Build history of the part. All positions in model axes, mm. Round coordinates to 2 decimals unless told otherwise and drop trailing zeros. Write each loop counter-clockwise with the first axis right and the second up, starting at its lowest first coordinate (ties: lowest second). Pieces come first, ordered by that corner, then holes. Notation, with made-up numbers: (51.5, 28.25) - (99.5, 28.25) arc R14 cw to (99.5, 47.25) - close; hole circle Ø6 at (26.5, 46.25). An arc over 180 degrees is marked (long way). Answer as a JSON object with one key per item and string values. Group by question number.
Item 1: Flat gauge pin, fed straight in: pin 1 (8 mm diameter, centred on x = 17.5, y = 25.5, fed in from -Z). Where does the tip first touch, or does it go through?
Item 2: Two-plate mould, pull along Y, no slides. Class faces 1 (the cylindrical face through (25.577, 38.226, 0.74)), 2 (the flat face through (43, 41, 0)): +Y half, -Y half, draft (parallel to the pull), parting line (faces both ways), or undercut.
Item 3: Slice it at A-A, the plane y = 40. List the corners of the cut face in (x, z).
Item 4: Probe line 1 (Y direction, x = 26.5, z = 0.85); line 2 (X direction, y = 69, z = 0.55); line 3 (X direction, y = 54.5, z = 1.45). List the from-to ranges inside material, lowest first. Write a range as from..to.
Item 5: Slice it at B-B, the plane x = 26.5. List the corners of the cut face in (y, z), then the cut area to 3 significant figures.
from build123d import *

# Parameters (mm, degrees)
SKETCH1_W           = 87.5
SKETCH1_H           = 80
BOSS_EXTRUDE1_DEPTH = 1.5
CUT_EXTRUDE1_DEPTH  = 80
SKETCH3_R           = 2
CUT_EXTRUDE2_DEPTH  = 1.5


with BuildPart() as part:
    # Sketch1 → Boss-Extrude1 (new body)
    with BuildSketch(Plane.XY):
        with Locations((43.75, 40)):
            Rectangle(SKETCH1_W, SKETCH1_H)
    extrude(amount=BOSS_EXTRUDE1_DEPTH)

    # Sketch2 → Cut-Extrude1 (cut)
    with BuildSketch(Plane(origin=(0, 80, 0), x_dir=(1, 0, 0), z_dir=(0, 1, 0))):
        Polygon((86.5, -0.492887182), (85.5, -0.492887182), (85.7, -1.5), (86.3, -1.5), align=None)
    extrude(amount=-CUT_EXTRUDE1_DEPTH, mode=Mode.SUBTRACT)

    # Sketch3 → Cut-Extrude2 (cut)
    with BuildSketch(Plane(origin=(0, 0, 0), x_dir=(-1, 0, 0), z_dir=(0, 0, -1))):
        with Locations((-26.5, 40)):
            Circle(SKETCH3_R)
    extrude(amount=-CUT_EXTRUDE2_DEPTH, mode=Mode.SUBTRACT)


solid = part.part
Geometry says:
{
 "1": {"pin 1": "stops at z = 0"},
 "2": {"face 1": "undercut", "face 2": "draft"},
 "3": {"outline": "(0, 0) - (24.5, 0) - (24.5, 1.5) - (0, 1.5) - close; (28.5, 0) - (87.5, 0) - (87.5, 1.5) - (86.3, 1.5) - (86.5, 0.49) - (85.5, 0.49) - (85.7, 1.5) - (28.5, 1.5) - close"},
 "4": {"line 1": "y = 0..38, 42..80", "line 2": "x = 0..85.51, 86.49..87.5", "line 3": "x = 0..85.69, 86.31..87.5"},
 "5": {"outline": "(0, 0) - (38, 0) - (38, 1.5) - (0, 1.5) - close; (42, 0) - (80, 0) - (80, 1.5) - (42, 1.5) - close", "area": "114 mm^2"}
}
